CAD build for the part. Positions are in the model's coordinates, mm. A direction names the side the tool comes from. Coordinates: 2 decimals unless noted, no trailing zeros. Order: outer loops, then holes, each group sorted by start corner. A loop starts at its lowest first (then second) coordinate and runs counter-clockwise, first axis right, second up. Notation, with made-up numbers: M -31.5,4 L 6.5,4 A16 ccw 6.5,24 Z; hole C 43.5,-27 d4. An arc over 180 degrees is marked long. One line per item, written item: value.
Autodesk Inventor part; units mm, degrees
ref_plane "YZ Plane" through (0, 0, 0) normal (1, 0, 0) x (0, 1, 0)
ref_plane "XZ Plane" through (0, 0, 0) normal (0, 1, 0) x (-1, 0, 0)
ref_plane "XY Plane" through (0, 0, 0) normal (0, 0, 1) x (1, 0, 0)
sketch "Sketch1" plane through (0, 0, 0) normal (0, 1, 0) x (-1, 0, 0)
  circle A0 centre (0, 0) radius 2.5
  circle A1 centre (0, 0) radius 3
  line L0 (1.9875, 0.25) -> (2.4875, 0.25)
  line L1 (2.4875, 0.25) -> (2.4875, -0.25)
  line L2 (2.4875, -0.25) -> (1.9875, -0.25)
  line L3 (1.9875, -0.25) -> (1.9875, 0.25)
  line L4 (1.9875, 0.25) -> (2.4875, -0.25) construction
  line L5 (2.4875, 0.25) -> (1.9875, -0.25) construction
  line L6 (2.5, 0) -> (-2.5, 0)
  line L7 (0.9958, 0.25) -> (0.9958, -0.25)
  line L8 (0.4958, 0.25) -> (0.9958, 0.25)
  line L9 (0.4958, -0.25) -> (0.4958, 0.25)
  line L10 (0.9958, -0.25) -> (0.4958, -0.25)
  line L11 (0.9958, 0.25) -> (0.4958, -0.25) construction
  line L12 (0.4958, 0.25) -> (0.9958, -0.25) construction
  line L13 (-0.4958, 0.25) -> (-0.4958, -0.25)
  line L14 (-0.9958, 0.25) -> (-0.4958, 0.25)
  line L15 (-0.9958, -0.25) -> (-0.9958, 0.25)
  line L16 (-0.4958, -0.25) -> (-0.9958, -0.25)
  line L17 (-0.4958, 0.25) -> (-0.9958, -0.25) construction
  line L18 (-0.9958, 0.25) -> (-0.4958, -0.25) construction
  line L19 (-1.9875, 0.25) -> (-1.9875, -0.25)
  line L20 (-2.4875, 0.25) -> (-1.9875, 0.25)
  line L21 (-2.4875, -0.25) -> (-2.4875, 0.25)
  line L22 (-1.9875, -0.25) -> (-2.4875, -0.25)
  line L23 (-1.9875, 0.25) -> (-2.4875, -0.25) construction
  line L24 (-2.4875, 0.25) -> (-1.9875, -0.25) construction
  point P0 (1.6583, 2.5)
  point P1 (-1.6583, 2.5)
  point P2 (2.2375, 0)
  point P3 (0.7458, 0)
  point P4 (-0.7458, 0)
  point P5 (-2.2375, 0)
  dimension "d11" = 5
  dimension "d12" = 0.5
  dimension "d22" = 1.4916
extrude "Extrusion3" add sketch "Sketch1" along normal blind 9 contours L6 L1 A0 | A0 L1 L6 | L0 L3 L6 L7 L8 L9 L13 L14 L15 L19 L20 A0 | L1 L6 L3 L0 | L2 L3 L6 L1 | A0 L22 L19 L6 L15 L16 L13 L9 L10 L7 L3 L2 | L21 L6 A0 | L20 L19 L6 L21 | A0 L6 L21 | L21 L6 L19 L22 | L7 L10 L9 L6 | L6 L9 L8 L7 | L15 L14 L13 L6 | L6 L13 L16 L15
extrude "Extrusion4" add sketch "Sketch1" along normal blind 0.5
fillet "Fillet2" radius 2.5 1 edges at (2.5, 9, 0)
extrude "Extrusion5" add sketch "Sketch1" against normal blind 24.5 contours L1 L6 L3 L0 | L2 L3 L6 L1 | L20 L19 L6 L21 | L21 L6 L19 L22 | L7 L10 L9 L6 | L6 L9 L8 L7 | L15 L14 L13 L6 | L6 L13 L16 L15
properties part number "ESP32_C3_SM" material "ABS Plastic"
Q1. Slice it at C-C (z = -1.3). List the corners of the cut face in (x, y), plus the area to 3 significant figures.
Recorded:
outline: M -2.7,0 L 2.7,0 L 2.7,0.5 L 2.14,0.5 L 2.14,6.5 A2.14 ccw -2.14,6.5 L -2.14,0.5 L -2.7,0.5 Z
area: 35.5 mm^2
Q2. Drill centre lines: line 1 along X through (y, z) = (-16, 0.15); line 2 along Y through (x, z) = (0.55, -2.7); line 3 along X through (y, z) = (2.5, -0.05). Where is each one in solid material? Low to high.
Recorded:
line 1: x = -2.49 to -1.99, -1 to -0.5, 0.5 to 1, 1.99 to 2.49
line 2: y = 0 to 0.5
line 3: x = -2.5 to 2.5
Q3. Which spindle directions (+Z, -Z, +X, -X, +Y, -Y) get a long thin tool onto all of the face, cutting with end or side? Do faces 1 (the face through (3, 0.2, -0.1)), 2 (the face through (2, 0.5, 2)). Say none if no direction does.
Recorded:
face 1: +Y, -Y
face 2: +Y
Q4. Pin check, flat tips, straight feed: pin 1 Ø1 at (y, z) = (-12.5, 1.5) entering from -X; pin 2 Ø3 at (y, z) = (-3.5, 0) entering from -X; pin 3 Ø0.6 at (x, y) = (-0.5, -17.5) entering from -Z; pin 4 Ø1.5 at (y, z) = (-8, 0.5) entering from +X. Stop position of each tip, or through.
Recorded:
pin 1: passes through
pin 2: stops at x = -2.49
pin 3: stops at z = -0.25
pin 4: stops at x = 2.49
Q5. Slice it at D-D (y = 1). List the corners of the cut face in (x, z), plus the area to 3 significant figures.
Recorded:
outline: C 0,0 d5
area: 19.6 mm^2
Q6. Slice it at A-A (y = -13.5). List the corners of the cut face in (x, z), plus the area to 4 significant figures.
Recorded:
outline: M -2.49,-0.25 L -1.99,-0.25 L -1.99,0.25 L -2.49,0.25 Z; M -1,-0.25 L -0.5,-0.25 L -0.5,0.25 L -1,0.25 Z; M 0.5,-0.25 L 1,-0.25 L 1,0.25 L 0.5,0.25 Z; M 1.99,-0.25 L 2.49,-0.25 L 2.49,0.25 L 1.99,0.25 Z
area: 1.000 mm^2
Q7. Slice it at B-B (x = 0). List the corners of the cut face in (y, z).
Recorded:
outline: M 0,-3 L 0.5,-3 L 0.5,-2.5 L 6.5,-2.5 A2.5 ccw 6.5,2.5 L 0.5,2.5 L 0.5,3 L 0,3 Z
